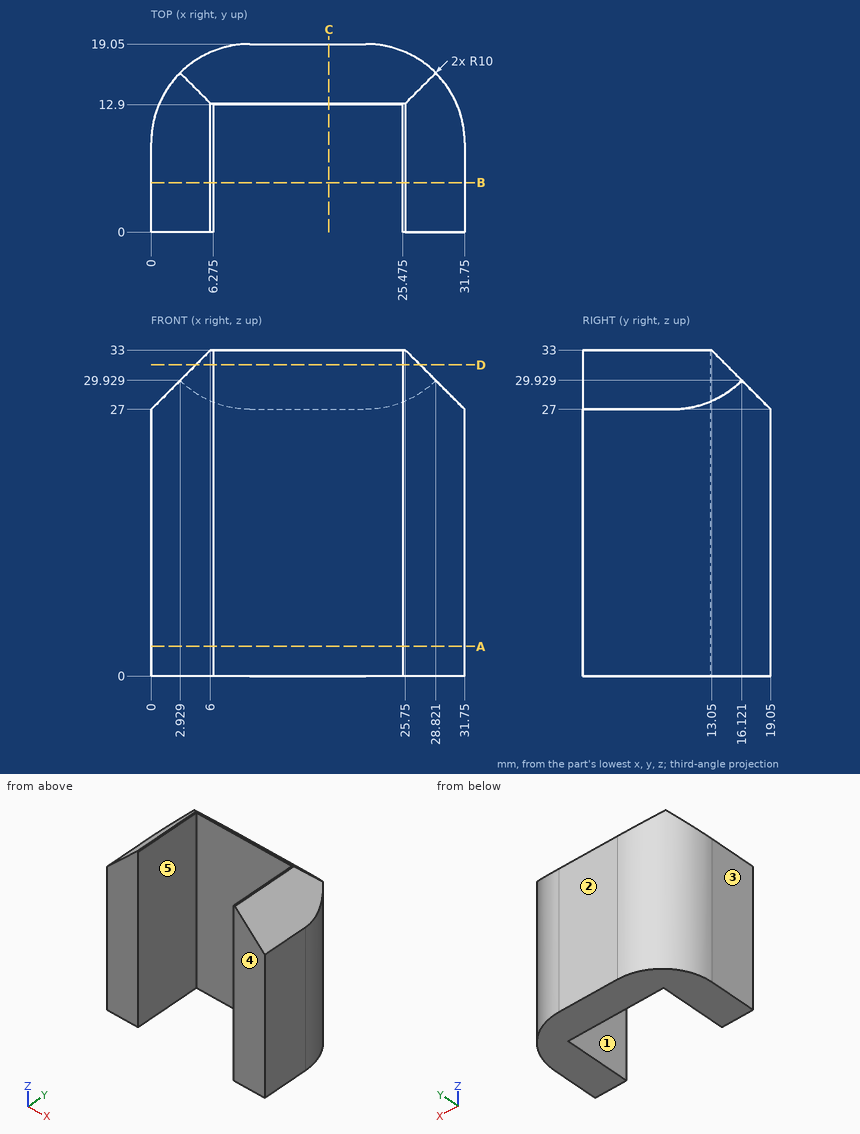
Part print with two shaded views. Sizes in mm from the minimum x, y, z corner. A direction names the side the tool comes from. Coordinates: 2 decimals unless noted, no trailing zeros. Loops run counter-clockwise (first coordinate to the right, second up) from the corner with the lowest first, then second, coordinate; pieces in that order, holes last. Notation, with made-up numbers: (-14.5, 3) -> (-7.5, 3) arc R29 cw to (-7.5, 28) -> close; hole circle Ø4 at (35.25, 46). An arc over 180 degrees is marked (long way). Answer as a JSON object with one key per item and string values.
Q1. Probe probe 1 along X at (y, z) = (5, 23) (3 decimals); probe 2 along X at (y, z) = (9.5, 22.5) (3 decimals); probe 3 along Y at (x, z) = (12, 15). List the from-to ranges inside material, lowest first.
Report:
{"probe 1": "x = 0 to 6.275, 25.475 to 31.75", "probe 2": "x = 0.01 to 6.275, 25.475 to 31.74", "probe 3": "y = 12.9 to 19.05"}
Q2. Cut at B-B (y = 5). List the corners of the cut face in (x, z) (3 decimals), and give its area (3 significant figures).
Report:
{"outline": "(0, 0) -> (6.275, 0) -> (6.275, 33) -> (6, 33) -> (0, 27) -> close; (25.475, 0) -> (31.75, 0) -> (31.75, 27) -> (25.75, 33) -> (25.475, 33) -> close", "area": "378 mm2"}
Q3. 3-axis set-ups, long thin cutter, end or side, ignore diameter. For the marked faces 1 and 2: which of +Z, -Z, +X, -X, +Y, -Y reach the whole face in a straight line?
Report:
{"face 1": "+Z, -Z, -Y", "face 2": "+Z, -Z, +X, -X, +Y"}
Q4. Pull direction X, two halves, no side cores. Call the marked faces 3, 4 and 5: released by +X, released by -X, zero draft, split by the parting line, or undercut.
Report:
{"face 3": "released by -X", "face 4": "zero draft", "face 5": "undercut"}
Q5. Flat gauge pins, fed straight in: P1, Ø5, axis at x = 10, z = 22.5, coming from the -Y side; P2, Ø8, axis at x = 24.5, y = 7.5, coming from the +Z side; P3, Ø2, axis at y = 12.5, z = 26.5, coming from the +X side; P4, Ø1.5, axis at x = 25.5, z = 13.5, coming from the +Y side. Where does each tip first touch, or does it go through?
Report:
{"P1": "stops at y = 12.9", "P2": "stops at z = 33", "P3": "stops at x = 31.45", "P4": "stops at y = 18.59"}
Q6. Cut at D-D (z = 31.5). List the corners of the cut face in (x, y) (3 decimals).
Report:
{"outline": "(4.5, 0) -> (6.275, 0) -> (6.275, 12.9) -> (25.475, 12.9) -> (25.475, 0) -> (27.25, 0) -> (27.25, 14.55) -> (4.5, 14.55) -> close"}
Q7. Cut at C-C (x = 18). List the corners of the cut face in (y, z), and give its area (3 significant figures).
Report:
{"outline": "(12.9, 0) -> (19.05, 0) -> (19.05, 27) -> (13.05, 33) -> (12.9, 33) -> close", "area": "185 mm2"}
Q8. Cut at A-A (z = 3). List the corners of the cut face in (x, y) (3 decimals).
Report:
{"outline": "(0, 0) -> (6.275, 0) -> (6.275, 12.9) -> (25.475, 12.9) -> (25.475, 0) -> (31.75, 0) -> (31.75, 9.05) arc R10 ccw to (21.75, 19.05) -> (10, 19.05) arc R10 ccw to (0, 9.05) -> close"}
